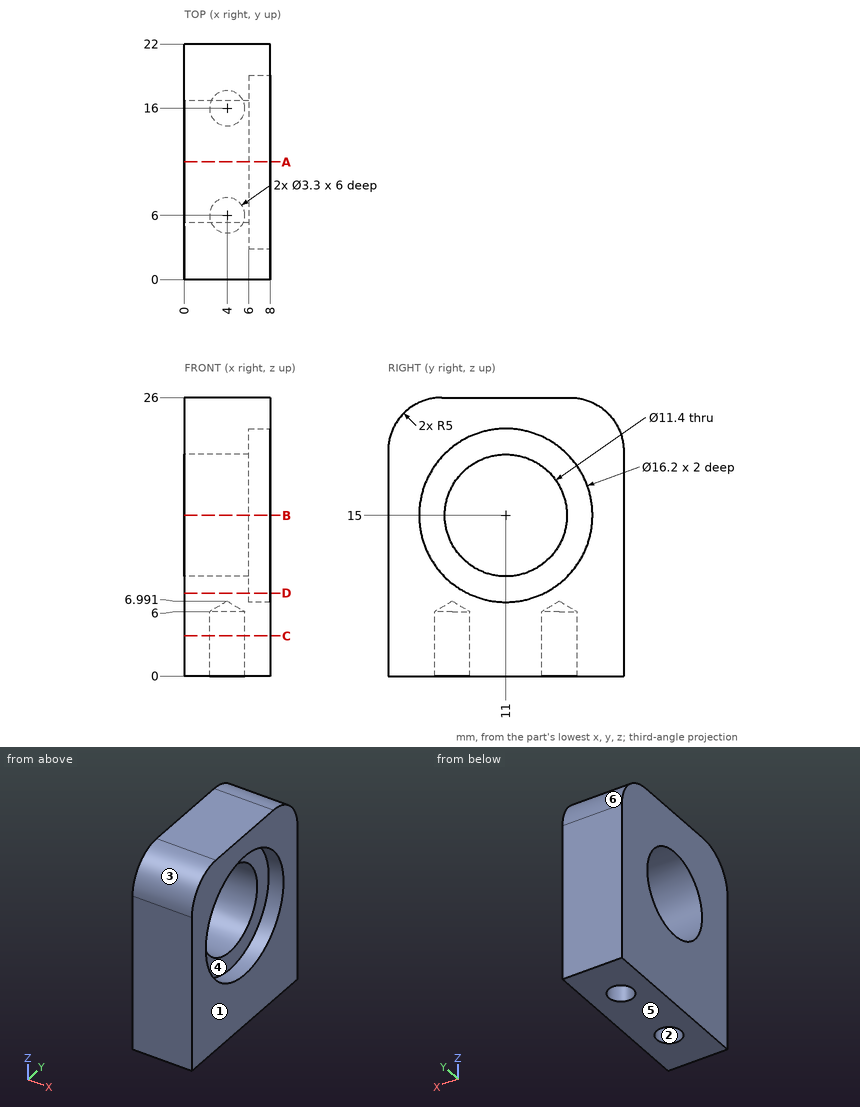
Part print with two shaded views. Sizes in mm from the minimum x, y, z corner. A direction names the side the tool comes from. Coordinates: 2 decimals unless noted, no trailing zeros. Write each loop counter-clockwise with the first axis right and the second up, starting at its lowest first coordinate (ties: lowest second). Pieces come first, ordered by that corner, then holes. Notation, with made-up numbers: (-13.75, 41.25) - (27.25, 41.25) arc R11 ccw to (27.25, 47.25) - close; hole circle Ø8 at (35.5, 47). An arc over 180 degrees is marked (long way). One line per item, written item: value. Start each with the question number.
1. Slice it at B-B (z = 15). Write the cut outline in (x, y).
2. Flat gauge pin, fed straight in: pin 1 (1.5 mm diameter, centred on x = 5.5, y = 20, fed in from +Z) (1 decimal). Where does the tip first touch, or does it go through?
3. Probe line 1 (Y direction, x = 4, z = 3.1); line 2 (Y direction, x = 7.45, z = 15); line 3 (Y direction, x = 5.25, z = 14.75) (1 decimal). List the from-to ranges inside material, lowest first. Write a range as from..to.
4. Slice it at D-D (z = 7.75). Write the cut outline in (x, y).
5. Slice it at A-A (y = 11). Write the cut outline in (x, z).
6. Mould opens along Y. For the marked faces 3, 4, 5 and 6 say: released by +Y, released by -Y, zero draft, split by the parting line, or undercut.
7. Slice it at C-C (z = 3.75). Write the cut outline in (x, y).
8. Tool access for the marked faces 1 and 2: list every direction of +Z, -Z, +X, -X, +Y, -Y with a clear straight run to the whole face (end or side of a thin tool).
Answers below:
1. outline: (0, 0) - (8, 0) - (8, 2.9) - (6, 2.9) - (6, 5.3) - (0, 5.3) - close; (0, 16.7) - (6, 16.7) - (6, 19.1) - (8, 19.1) - (8, 22) - (0, 22) - close
2. pin 1: stops at z = 25.5
3. line 1: y = 0..4.35, 7.65..14.35, 17.65..22
3. line 2: y = 0..2.9, 19.1..22
3. line 3: y = 0..5.3, 16.7..22
4. outline: (0, 0) - (8, 0) - (8, 7.39) - (6, 7.39) - (6, 14.61) - (8, 14.61) - (8, 22) - (0, 22) - close
5. outline: (0, 0) - (8, 0) - (8, 6.9) - (6, 6.9) - (6, 9.3) - (0, 9.3) - close; (0, 20.7) - (6, 20.7) - (6, 23.1) - (8, 23.1) - (8, 26) - (0, 26) - close
6. face 3: released by -Y
6. face 4: undercut
6. face 5: zero draft
6. face 6: released by +Y
7. outline: (0, 0) - (8, 0) - (8, 22) - (0, 22) - close; hole circle Ø3.3 at (4, 6); hole circle Ø3.3 at (4, 16)
8. face 1: +Z, -Z, +X, +Y, -Y
8. face 2: -Z
